from build123d import *

# Parameters (mm, degrees)
SKETCH1_W               = 27
SKETCH1_H               = 18.05
SKETCH1_W_2             = 15
SKETCH1_H_2             = 30
SKETCH1_H_3             = 25
BOSS_EXTRUDE1_DEPTH     = 59.5
SKETCH3_W               = 15
SKETCH3_H               = 75
CUT_EXTRUDE2_DEPTH      = 53.95
SKETCH4_W               = 6
SKETCH4_H               = 16.6
SKETCH4_H_2             = 21.6
CUT_EXTRUDE3_DEPTH      = 10
CUT_EXTRUDE4_DEPTH      = 1
CUT_EXTRUDE4_DEPTH_BACK = 54
CUT_EXTRUDE5_DEPTH      = 1
CUT_EXTRUDE5_DEPTH_BACK = 17.2
SKETCH8_W               = 42.3
SKETCH8_H               = 3.8
CUT_EXTRUDE6_DEPTH      = 51.9
CUT_EXTRUDE7_DEPTH      = 16
CUT_EXTRUDE7_DEPTH_BACK = 60
CUT_EXTRUDE8_DEPTH      = 60


with BuildPart() as part:
    # Sketch1 → Boss-Extrude1 (new body)
    with BuildSketch(Plane.XY):
        Polygon((71.3, 0), (15, 0), (15, 25), (15, 75), (71.3, 75), align=None)
        with Locations((42.6, 35.225)):
            Rectangle(SKETCH1_W, SKETCH1_H, mode=Mode.SUBTRACT)
        with Locations((78.8, 60)):
            Rectangle(SKETCH1_W_2, SKETCH1_H_2)
        with Locations((78.8, 12.5)):
            Rectangle(SKETCH1_W_2, SKETCH1_H_3)
        with Locations((7.5, 12.5)):
            Rectangle(SKETCH1_W_2, SKETCH1_H_3)
        with Locations((7.5, 60)):
            Rectangle(SKETCH1_W_2, SKETCH1_H_2)
    extrude(amount=BOSS_EXTRUDE1_DEPTH)

    # Sketch3 → Cut-Extrude2 (cut)
    with BuildSketch(Plane.XY.offset(59.5)):
        with Locations((7.5, 37.5)):
            Rectangle(SKETCH3_W, SKETCH3_H)
        with Locations((78.8, 37.5)):
            Rectangle(SKETCH3_W, SKETCH3_H)
    extrude(amount=-CUT_EXTRUDE2_DEPTH, mode=Mode.SUBTRACT)

    # Sketch4 → Cut-Extrude3 (cut)
    with BuildSketch(Plane.XY.offset(5.55)):
        with Locations((7.7, 12.5)):
            Rectangle(SKETCH4_W, SKETCH4_H)
        with Locations((7.7, 60)):
            Rectangle(SKETCH4_W, SKETCH4_H_2)
        with Locations((78.6, 60)):
            Rectangle(SKETCH4_W, SKETCH4_H_2)
        with Locations((78.6, 12.5)):
            Rectangle(SKETCH4_W, SKETCH4_H)
    extrude(amount=-CUT_EXTRUDE3_DEPTH, mode=Mode.SUBTRACT)

    # Sketch6 → Cut-Extrude4 (cut, two sides)
    with BuildSketch(Plane(origin=(0, 75, 0), x_dir=(1, 0, 0), z_dir=(0, 1, 0))) as cut_extrude4_sk:
        Polygon((18, 191.164455675), (18, 0), (18, -55.9), (68.3, -55.9), (68.3, 0), (68.3, 191.164455675), (68.3, 573.493367025), (18, 573.493367025), align=None)
    extrude(amount=CUT_EXTRUDE4_DEPTH, mode=Mode.SUBTRACT)
    extrude(cut_extrude4_sk.sketch, amount=-CUT_EXTRUDE4_DEPTH_BACK, mode=Mode.SUBTRACT)

    # Sketch7 → Cut-Extrude5 (cut, two sides)
    with BuildSketch(Plane.XZ) as cut_extrude5_sk:
        Polygon((18, -191.164455675), (18, 0), (18, 55.9), (68.3, 55.9), (68.3, 0), (68.3, -191.164455675), (68.3, -573.493367025), (18, -573.493367025), align=None)
    extrude(amount=CUT_EXTRUDE5_DEPTH, mode=Mode.SUBTRACT)
    extrude(cut_extrude5_sk.sketch, amount=-CUT_EXTRUDE5_DEPTH_BACK, mode=Mode.SUBTRACT)

    # Sketch8 → Cut-Extrude6 (cut)
    with BuildSketch(Plane(origin=(0, 0, 0), x_dir=(-1, 0, 0), z_dir=(0, 0, -1))):
        with Locations((-43.15, 19.1)):
            Rectangle(SKETCH8_W, SKETCH8_H)
    extrude(amount=-CUT_EXTRUDE6_DEPTH, mode=Mode.SUBTRACT)

    # Sketch9 → Cut-Extrude7 (cut, two sides)
    with BuildSketch(Plane.ZY.offset(-15)) as cut_extrude7_sk:
        Polygon((-165.43809057, 45), (0, 45), (38.5, 45), (38.5, 25), (0, 25), (-165.43809057, 25), (-496.31427171, 25), (-496.31427171, 45), align=None)
    extrude(amount=CUT_EXTRUDE7_DEPTH, mode=Mode.SUBTRACT)
    extrude(cut_extrude7_sk.sketch, amount=-CUT_EXTRUDE7_DEPTH_BACK, mode=Mode.SUBTRACT)

    # Sketch11 → Cut-Extrude8 (cut)
    with BuildSketch(Plane(origin=(71.3, 0, 0), x_dir=(0, 0, -1), z_dir=(1, 0, 0))):
        Polygon((-5.55, 0), (-59.5, 17.2), (-59.5, 0), align=None)
    extrude(amount=-CUT_EXTRUDE8_DEPTH, mode=Mode.SUBTRACT)


solid = part.part
Check sheet for the modelled part. Datum: model origin and axes. Units: mm. A direction names the side the tool comes from. Coordinates: 2 decimals unless noted, no trailing zeros. Write each loop counter-clockwise with the first axis right and the second up, starting at its lowest first coordinate (ties: lowest second). Pieces come first, ordered by that corner, then holes. Notation, with made-up numbers: M 45.5,50 L 72.5,50 A12 ccw 72.5,73 Z; hole C -27.75,54.5 d8. An arc over 180 degrees is marked long. Answer as CSV lines item,"result".
Q1. Cross-section at C-C (z = 44). Record the boundary of the cut face in (x, y), then the cut area to 3 significant figures.
Check result:
outline,"M 15,12.26 L 18,12.26 L 18,17.2 L 22,17.2 L 22,21 L 18,21 L 18,75 L 15,75 Z; M 64.3,17.2 L 68.3,17.2 L 68.3,12.26 L 71.3,12.26 L 71.3,75 L 68.3,75 L 68.3,21 L 64.3,21 Z"
area,"407 mm^2"
Q2. Material ranges on probe 1 along X at (y, z) = (52.5, 22); probe 2 along Z at (x, y) = (67, 56.5); probe 3 along Z at (x, y) = (71, 37), recorded low to high. Write a range as from..to.
Check result:
probe 1,"15..18, 68.3..71.3"
probe 2,"55.9..59.5"
probe 3,"38.5..59.5"
Q3. Cross-section at B-B (x = 40.5). Record the boundary of the cut face in (y, z).
Check result:
outline,"M 16.05,55.9 L 17.2,55.9 L 17.2,51.9 L 21,51.9 L 21,55.9 L 26.2,55.9 L 26.2,59.5 L 17.2,59.5 Z; M 44.25,55.9 L 75,55.9 L 75,59.5 L 44.25,59.5 Z"
Q4. Cross-section at A-A (y = 67). Record the boundary of the cut face in (x, z), then the cut area to 3 significant figures.
Check result:
outline,"M 0,0 L 4.7,0 L 4.7,5.55 L 0,5.55 Z; M 10.7,0 L 18,0 L 18,55.9 L 68.3,55.9 L 68.3,0 L 75.6,0 L 75.6,5.55 L 71.3,5.55 L 71.3,59.5 L 15,59.5 L 15,5.55 L 10.7,5.55 Z; M 81.6,0 L 86.3,0 L 86.3,5.55 L 81.6,5.55 Z"
area,"638 mm^2"
Q5. Cross-section at D-D (y = 42). Record the boundary of the cut face in (x, z), then the cut area to 3 significant figures.
Check result:
outline,"M 15,38.5 L 18,38.5 L 18,55.9 L 29.1,55.9 L 29.1,59.5 L 15,59.5 Z; M 56.1,55.9 L 68.3,55.9 L 68.3,38.5 L 71.3,38.5 L 71.3,59.5 L 56.1,59.5 Z"
area,"210 mm^2"
Q6. Set-up check for faces 1 (the face through (16, 25, 12)), 2 (the face through (18, 54, 28)), 3 (the face through (79, 70.8, 3)), 4 (the face through (4, 13, 5.55)): record each of +Z, -Z, +X, -X, +Y, -Y from which the full face is reachable in a straight line by a thin tool's end or side.
Check result:
face 1,"-Z, +X, -X"
face 2,"-Z, +Y"
face 3,"+Z, -Z"
face 4,"+Z, -X, +Y, -Y"
Q7. Go/stop test with flat-tipped pins: pin 1 (1.9 mm diameter, centred on x = 41.5, y = 18.5, fed in from -Z); pin 2 (19 mm diameter, centred on y = 9, z = 24, fed in from -X); pin 3 (7.5 mm diameter, centred on x = 7.5, y = 7.5, fed in from +Z); pin 4 (6 mm diameter, centred on x = 47.5, y = 38.5, fed in from +Z). Record where each tip stops, or that it passes through.
Check result:
pin 1,"z = 51.9"
pin 2,"x = 15"
pin 3,"z = 5.55"
pin 4,"through"
Q8. Mould release check, pull along X, two halves, no side actions. Record for faces 5 (the face through (0, 12, 3)), 6 (the face through (9, 0, 3)), 7 (the face through (43, 21, 53)), 8 (the face through (71.3, 45.3, 32.9)): released by +X, released by -X, zero draft, split by the parting line, or undercut.
Check result:
face 5,"released by -X"
face 6,"zero draft"
face 7,"undercut"
face 8,"released by +X"
